Here's how the part is built. I have some questions about the finished solid (model axes, mm). A direction names the side the tool comes from. Coordinates: 2 decimals unless noted, no trailing zeros. Write each loop counter-clockwise with the first axis right and the second up, starting at its lowest first coordinate (ties: lowest second). Pieces come first, ordered by that corner, then holes. Notation, with made-up numbers: M 28.5,71 L 45.5,71 A16 ccw 45.5,102 Z; hole C 67,17.5 d2. An arc over 180 degrees is marked long. Write each question's results on one line, items separated by ' | '. Start each with the question number.
from build123d import *

# Parameters (mm, degrees)
BOSS_EXTRUDE1_DEPTH = 27
BOSS_EXTRUDE2_DEPTH = 2
SKETCH3_R           = 2.1
CUT_EXTRUDE1_DEPTH  = 37.084103148
SKETCH4_R           = 1.4
CUT_EXTRUDE2_DEPTH  = 37.084103148
FILLET1_R           = 1
FILLET2_R           = 4
SKETCH5_R           = 0.75
CUT_EXTRUDE3_DEPTH  = 36.06600926


with BuildPart() as part:
    # Sketch1 → Boss-Extrude1 (new body)
    with BuildSketch(Plane.XY):
        Polygon((7.5, -4.75), (-7.5, -4.75), (-7.5, 0), (-13.75, 0), (-13.75, -10), (13.75, -10), (13.75, 0), (7.5, 0), align=None)
    extrude(amount=BOSS_EXTRUDE1_DEPTH)

    # Sketch2 → Boss-Extrude2 (add)
    with BuildSketch(Plane.XZ.offset(10)):
        with BuildLine():
            Line((13.75, 21.5), (13.75, 5.5))
            ThreePointArc((13.75, 5.5), (21.75, 13.5), (13.75, 21.5))
        make_face()
        with BuildLine():
            Line((-13.75, 21.5), (-13.75, 5.5))
            ThreePointArc((-13.75, 5.5), (-21.75, 13.5), (-13.75, 21.5))
        make_face()
    extrude(amount=-BOSS_EXTRUDE2_DEPTH)

    # Sketch3 → Cut-Extrude1 (cut, through all)
    with BuildSketch(Plane(origin=(0, 0, 0), x_dir=(1, 0, 0), z_dir=(0, 1, 0))):
        with Locations(Location((-10.625, -20, 0), (0, 0, 270))):
            Circle(SKETCH3_R)
        with Locations(Location((10.625, -20, 0), (0, 0, 270))):
            Circle(SKETCH3_R)
        with Locations(Location((-10.625, -7, 0), (0, 0, 270))):
            Circle(SKETCH3_R)
        with Locations(Location((10.625, -7, 0), (0, 0, 270))):
            Circle(SKETCH3_R)
    extrude(amount=-CUT_EXTRUDE1_DEPTH, mode=Mode.SUBTRACT)

    # Sketch4 → Cut-Extrude2 (cut, through all)
    with BuildSketch(Plane.XY.offset(27)):
        with Locations((0, -7.375)):
            Circle(SKETCH4_R)
    extrude(amount=-CUT_EXTRUDE2_DEPTH, mode=Mode.SUBTRACT)

    # Fillet1
    fillet1_edges = [part.edges().sort_by_distance(p)[0] for p in [
        (-7.5, -4.75, 13.5),
        (7.5, -4.75, 13.5),
    ]]
    fillet(fillet1_edges, radius=FILLET1_R)

    # Fillet2
    fillet2_edges = [part.edges().sort_by_distance(p)[0] for p in [
        (13.75, -9, 21.5),
        (13.75, -8, 13.5),
        (13.75, -9, 5.5),
        (-13.75, -9, 5.5),
        (-13.75, -8, 13.5),
        (-13.75, -9, 21.5),
    ]]
    fillet(fillet2_edges, radius=FILLET2_R)

    # Sketch5 → Cut-Extrude3 (cut, through all)
    with BuildSketch(Plane(origin=(0, -4.75, 0), x_dir=(1, 0, 0), z_dir=(0, 1, 0))):
        with Locations(Location((3.5, -6, 0), (0, 0, 180))):
            Circle(SKETCH5_R)
        with Locations(Location((-3.5, -21, 0), (0, 0, 180))):
            Circle(SKETCH5_R)
    extrude(amount=-CUT_EXTRUDE3_DEPTH, mode=Mode.SUBTRACT)


solid = part.part
1) Please list where these lines run through material, in increasing order: line 1 (X direction, y = -2.25, z = 20) (3 decimals); line 2 (Z direction, x = -9, y = -7.75); line 3 (X direction, y = -7.25, z = 1.75). Write a range as [from, to].
2) I want a section at C-C, the plane z = 13. Write out the boundary of the cut face in (x, y) (3 decimals), then the cut area to 3 significant figures.
3) I want a section at B-B, the plane y = -2. Write out the boundary of the cut face in (x, z) (3 decimals).
4) For pin 1 Ø3.5 at (x, z) = (-10.625, 7) entering from -Y; pin 2 Ø5 at (y, z) = (-6, 16.5) entering from -X; pin 3 Ø5 at (x, z) = (-2.5, 15.5) entering from +Y; pin 4 Ø4 at (y, z) = (-2, 17.5) entering from -X, each with a flat end and sliding along its axis, tell me the tip position at first contact or that it passes through.
5) For faces 1 (the cylindrical face through (14.891, -6.797, 13.342)), 2 (the flat face through (-19, -8, 14)), 3 (the flat face through (0, -4.75, 13)), which set-ups out of +Z, -Z, +X, -X, +Y, -Y let a thin tool reach every point of the face, with its end or its side?
6) We'd pull the mould along Z, two halves only. Please class faces 4 (the cylindrical face through (21.75, -9.15, 13.36)), 5 (the cylindrical face through (12.04, -4.93, 5.45)), 6 (the cylindrical face through (14.184, -7.625, 3.998)), 7 (the flat face through (-11, 0, 13)): pulls with the +Z half, pulls with the -Z half, needs draft (parallel to the pull), parting line crosses it, or undercut.
7) I want a section at A-A, the plane x = 3.5. Write out the boundary of the cut face in (y, z), then the cut area to 3 significant figures.
Output:
1) line 1: x = [-13.75, -12.725], [-8.525, -7.5], [7.5, 8.525], [12.725, 13.75] | line 2: z = [0, 5.67], [8.33, 18.67], [21.33, 27] | line 3: x = [-13.75, -1.39], [1.39, 13.75]
2) outline: M -21.734,-10 L 21.734,-10 L 21.734,-8 L 17.75,-8 A4 cw 13.75,-4 L 13.75,0 L 7.5,0 L 7.5,-3.75 A1 cw 6.5,-4.75 L -6.5,-4.75 A1 cw -7.5,-3.75 L -7.5,0 L -13.75,0 L -13.75,-4 A4 cw -17.75,-8 L -21.734,-8 Z; hole C 0,-7.375 d2.8 | area: 237 mm2
3) outline: M -13.75,0 L -7.5,0 L -7.5,27 L -13.75,27 Z; M 7.5,0 L 13.75,0 L 13.75,27 L 7.5,27 Z; hole C -10.625,7 d4.2; hole C -10.625,20 d4.2; hole C 10.625,7 d4.2; hole C 10.625,20 d4.2
4) pin 1: passes through | pin 2: stops at x = -21.61 | pin 3: stops at y = -4.75 | pin 4: stops at x = -13.75
5) face 1: +Z, -Z, +X, +Y | face 2: +Z, -Z, -X, +Y | face 3: +Z, -Z, +Y
6) face 4: parting line crosses it | face 5: undercut | face 6: pulls with the -Z half | face 7: needs draft
7) outline: M -10,0 L -4.75,0 L -4.75,5.25 L -10,5.25 Z; M -10,6.75 L -4.75,6.75 L -4.75,27 L -10,27 Z | area: 134 mm2
